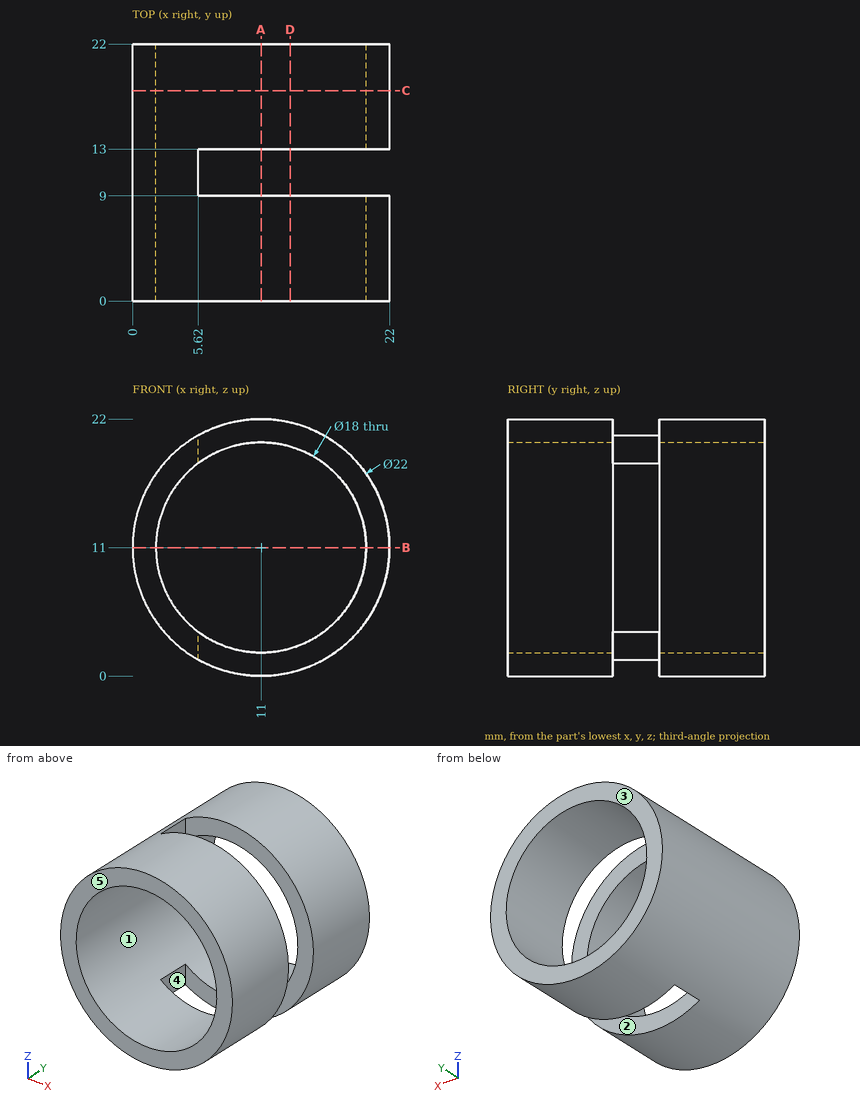
Part print with two shaded views. Sizes in mm from the minimum x, y, z corner. A direction names the side the tool comes from. Coordinates: 2 decimals unless noted, no trailing zeros. Write each loop counter-clockwise with the first axis right and the second up, starting at its lowest first coordinate (ties: lowest second). Pieces come first, ordered by that corner, then holes.
(1) 3-axis set-ups, long thin cutter, end or side, ignore diameter. For the marked faces 1 and 2: which of +Z, -Z, +X, -X, +Y, -Y reach the whole face in a straight line?
(2) Mould opens along Y. For the marked faces 3, 4 and 5 say: pulls with the +Y half, pulls with the -Y half, needs draft (parallel to the pull), parting line crosses it, or undercut.
(3) Drill centre lines: line 1 (Y direction, x = 16.25, z = 19.25); line 2 (X direction, y = 7.25, z = 11); line 3 (X direction, y = 19.75, z = 10). Where is each one in solid material? Low to high.
(4) Cut at D-D on x = 13.5. List the corners of the cut face in (y, z).
(5) Cut at A-A on x = 11. List the corners of the cut face in (y, z), and give its area (3 significant figures).
(6) Cut at B-B on z = 11. List the corners of the cut face in (x, y).
(7) Pin check, flat tips, straight feed: pin 1 Ø4 at (y, z) = (7.5, 15.5) entering from +X; pin 2 Ø0.7 at (y, z) = (11, 3) entering from +X; pin 3 Ø8 at (y, z) = (8, 16.5) entering from +X. Stop position of each tip, or through.
(8) Cut at C-C on y = 18. List the corners of the cut face in (x, z), and give its area (3 significant figures).
Working result:
1. face 1: +Y, -Y
1. face 2: +Z, -Z, +X
2. face 3: pulls with the +Y half
2. face 4: undercut
2. face 5: pulls with the -Y half
3. line 1: y = 0 to 9, 13 to 22
3. line 2: x = 0 to 2, 20 to 22
3. line 3: x = 0.05 to 2.06, 19.94 to 21.95
4. outline: (0, 0.29) - (9, 0.29) - (9, 2.35) - (0, 2.35) - close; (0, 19.65) - (9, 19.65) - (9, 21.71) - (0, 21.71) - close; (13, 0.29) - (22, 0.29) - (22, 2.35) - (13, 2.35) - close; (13, 19.65) - (22, 19.65) - (22, 21.71) - (13, 21.71) - close
5. outline: (0, 0) - (9, 0) - (9, 2) - (0, 2) - close; (0, 20) - (9, 20) - (9, 22) - (0, 22) - close; (13, 0) - (22, 0) - (22, 2) - (13, 2) - close; (13, 20) - (22, 20) - (22, 22) - (13, 22) - close
5. area: 72.0 mm2
6. outline: (0, 0) - (2, 0) - (2, 22) - (0, 22) - close; (20, 0) - (22, 0) - (22, 9) - (20, 9) - close; (20, 13) - (22, 13) - (22, 22) - (20, 22) - close
7. pin 1: stops at x = 21.71
7. pin 2: stops at x = 5.62
7. pin 3: stops at x = 21.9
8. outline: circle Ø22 at (11, 11); hole circle Ø18 at (11, 11)
8. area: 126 mm2
